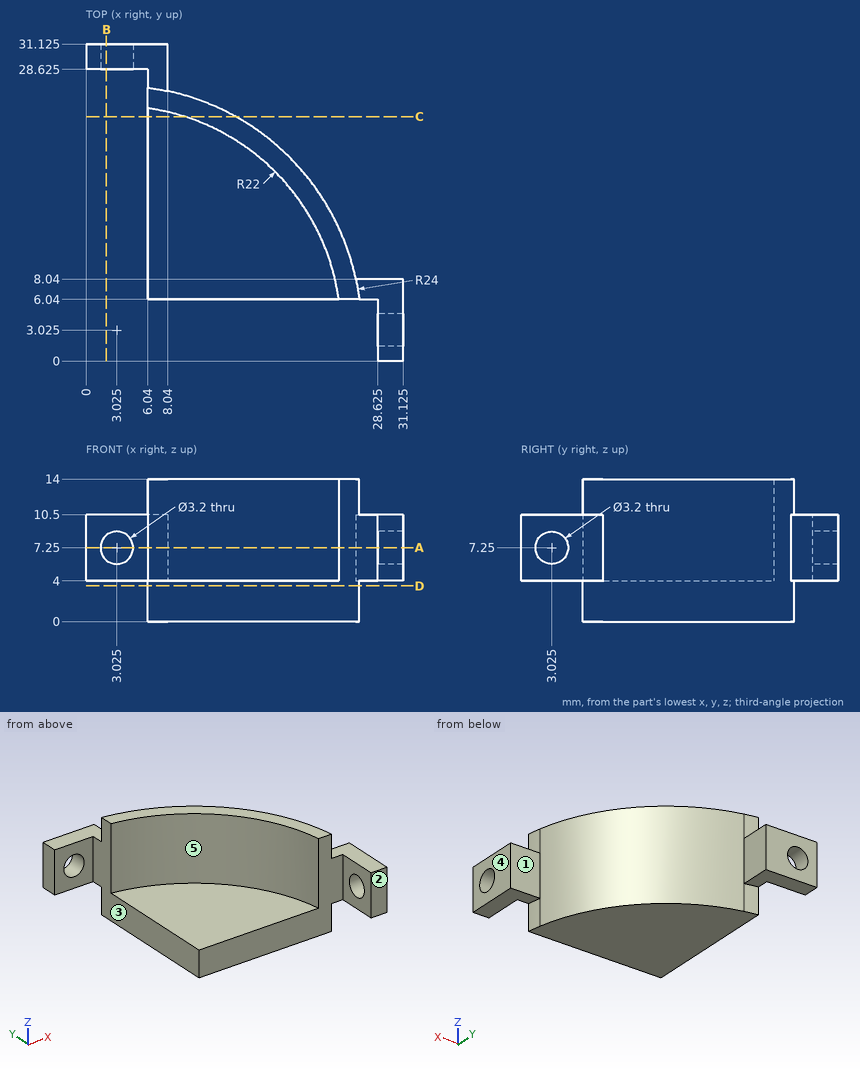
Source: three-view drawing plus pictorial views. Frame: mm from the lowest corner of the part. A direction names the side the tool comes from. Coordinates: 2 decimals unless noted, no trailing zeros. Order: outer loops, then holes, each group sorted by start corner. A loop starts at its lowest first (then second) coordinate and runs counter-clockwise, first axis right, second up. Notation, with made-up numbers: M -8,-9.75 L 38,-9.75 A16 ccw 38,-4.75 Z; hole C 50,-9 d3. An arc over 180 degrees is marked long. Answer in a Markdown table with one row per item.
(1) Access query for the marked faces 1, 2, 3, 4 and 5. Directions: +Z, -Z, +X, -X, +Y, -Y. A direction counts if a zero-diameter tool reaches every point of the face in a straight line with its end or side. Return the directions, or none.
Numbers:
| item | result |
|---|---|
| face 1 | +Z, -Z, +X, +Y |
| face 2 | +Z, -Z, +X, -X, -Y |
| face 3 | +Z, -Z, -X, -Y |
| face 4 | +Z, -Z, +X, +Y, -Y |
| face 5 | +Z, -X, -Y |
(2) Section query D-D, the plane z = 3.5. Output: boundary loops of the cut face in (x, y) (3 decimals), plus the area to 3 significant figures.
Numbers:
| item | result |
|---|---|
| outline | M 6.04,6.04 L 26.835,6.04 A24 ccw 6.04,26.835 Z |
| area | 317 mm^2 |
(3) Material intervals for line 1 (Y direction, x = 29.4, z = 7.25) (3 decimals); line 2 (Y direction, x = 30.5, z = 5); line 3 (Z direction, x = 9, y = 11), sorted ascending. Write a range as [from, to].
Numbers:
| item | result |
|---|---|
| line 1 | y = [0, 1.425], [4.625, 8.04] |
| line 2 | y = [0, 8.04] |
| line 3 | z = [0, 4] |
(4) Contact query for flat-ended pins moving along their axis: pin 1 Ø2 at (y, z) = (7.5, 2.5) entering from -X; pin 2 Ø10 at (x, y) = (14.5, 8) entering from +Z; pin 3 Ø3.5 at (x, y) = (3, 28.5) entering from -Z. Output: stop coordinate, or through.
Numbers:
| item | result |
|---|---|
| pin 1 | stops at x = 6.04 |
| pin 2 | stops at z = 4 |
| pin 3 | stops at z = 4 |
(5) Section query C-C, the plane y = 24. Output: boundary loops of the cut face in (x, z), plus the area to 3 significant figures.
Numbers:
| item | result |
|---|---|
| outline | M 6.04,0 L 14.69,0 L 14.69,14 L 9.66,14 L 9.66,4 L 6.04,4 Z |
| area | 84.9 mm^2 |
(6) Section query A-A, the plane z = 7.25. Output: boundary loops of the cut face in (x, y) (3 decimals).
Numbers:
| item | result |
|---|---|
| outline | M 0,28.625 L 1.425,28.625 L 1.425,31.125 L 0,31.125 Z; M 4.625,28.625 L 6.04,28.625 L 6.04,24.817 A22 cw 24.817,6.04 L 28.625,6.04 L 28.625,4.625 L 31.125,4.625 L 31.125,8.04 L 26.495,8.04 A24 ccw 8.04,26.495 L 8.04,31.125 L 4.625,31.125 Z; M 28.625,0 L 31.125,0 L 31.125,1.425 L 28.625,1.425 Z |
(7) Section query B-B, the plane x = 2. Output: boundary loops of the cut face in (y, z) (3 decimals).
Numbers:
| item | result |
|---|---|
| outline | M 28.625,4 L 31.125,4 L 31.125,6.021 L 28.625,6.021 Z; M 28.625,8.479 L 31.125,8.479 L 31.125,10.5 L 28.625,10.5 Z |
